Here's how the part is built. I have some questions about the finished solid (model axes, mm). A direction names the side the tool comes from. Round coordinates to 2 decimals unless told otherwise and drop trailing zeros. Write each loop counter-clockwise with the first axis right and the second up, starting at its lowest first coordinate (ties: lowest second). Pieces come first, ordered by that corner, then holes. Notation, with made-up numbers: (18, 79.25) -> (51, 79.25) arc R24 cw to (51, 115.25) -> close; hole circle Ø3 at (25.5, 65.5). An arc over 180 degrees is marked (long way). Answer in a Markdown table with one row per item.
from build123d import *

# Parameters (mm, degrees)
BOSS_EXTRUDE1_DEPTH = 7
FILLET1_R           = 2
SKETCH2_R           = 1.5
SKETCH2_R_2         = 1.1
BOSS_EXTRUDE2_DEPTH = 4
SKETCH3_R           = 1.5
SKETCH3_R_2         = 1.1
SKETCH3_W           = 4.5
SKETCH3_H           = 1.5
BOSS_EXTRUDE3_DEPTH = 4


with BuildPart() as part:
    # Sketch1 → Boss-Extrude1 (new body)
    with BuildSketch(Plane(origin=(0, 0, 0), x_dir=(1, 0, 0), z_dir=(0, 1, 0))):
        with BuildLine():
            Line((10, 9), (-10, 9))
            ThreePointArc((-10, 9), (-11.414213562, 8.414213562), (-12, 7))
            Line((-12, 7), (-12, -7))
            ThreePointArc((-12, -7), (-11.414213562, -8.414213562), (-10, -9))
            Line((-10, -9), (10, -9))
            ThreePointArc((10, -9), (11.414213562, -8.414213562), (12, -7))
            Line((12, -7), (12, 7))
            ThreePointArc((12, 7), (11.414213562, 8.414213562), (10, 9))
        make_face()
    extrude(amount=BOSS_EXTRUDE1_DEPTH)

    # Fillet1
    fillet1_edges = [part.edges().sort_by_distance(p)[0] for p in [
        (12, 0, 0),
        (11.414213562, 0, 8.414213562),
        (0, 0, 9),
        (-11.414213562, 0, 8.414213562),
        (11.414213562, 7, 8.414213562),
        (12, 7, 0),
        (11.414213562, 7, -8.414213562),
        (0, 7, -9),
        (-11.414213562, 7, -8.414213562),
        (-12, 7, 0),
        (-11.414213562, 7, 8.414213562),
        (-12, 0, 0),
        (0, 7, 9),
        (-11.414213562, 0, -8.414213562),
        (0, 0, -9),
        (11.414213562, 0, -8.414213562),
    ]]
    fillet(fillet1_edges, radius=FILLET1_R)

    # Sketch2 → Boss-Extrude2 (add)
    # profile 1 of 3: a face of its own
    with BuildSketch(Plane.ZY.offset(12)):
        with Locations(Location((0, 3.5, 0), (0, 0, 270))):
            Circle(SKETCH2_R)
        with Locations((0, 3.5)):
            Circle(SKETCH2_R_2, mode=Mode.SUBTRACT)
    # profile 2 of 3: a face of its own
    with BuildSketch(Plane.ZY.offset(12)):
        with Locations(Location((7, 3.5, 0), (0, 0, 270))):
            Circle(SKETCH2_R)
        with Locations(Location((7, 3.5, 0), (0, 0, 90))):
            Circle(SKETCH2_R_2, mode=Mode.SUBTRACT)
    # profile 3 of 3: a face of its own
    with BuildSketch(Plane.ZY.offset(12)):
        with Locations(Location((-7, 3.5, 0), (0, 0, 270))):
            Circle(SKETCH2_R)
        with Locations(Location((-7, 3.5, 0), (0, 0, 90))):
            Circle(SKETCH2_R_2, mode=Mode.SUBTRACT)
    extrude(amount=BOSS_EXTRUDE2_DEPTH)

    # Sketch3 → Boss-Extrude3 (add)
    # profile 1 of 3: a face of its own
    with BuildSketch(Plane(origin=(12, 0, 0), x_dir=(0, 0, -1), z_dir=(1, 0, 0))):
        with Locations(Location((-5.233431742, 3.5, 0), (0, 0, 270))):
            Circle(SKETCH3_R)
        with Locations((-5.233431742, 3.5)):
            Circle(SKETCH3_R_2, mode=Mode.SUBTRACT)
    # profile 2 of 3: a face of its own
    with BuildSketch(Plane(origin=(12, 0, 0), x_dir=(0, 0, -1), z_dir=(1, 0, 0))):
        with Locations(Location((-0.833431742, 3.5, 0), (0, 0, 270))):
            Circle(SKETCH3_R)
        with Locations((-0.833431742, 3.5)):
            Circle(SKETCH3_R_2, mode=Mode.SUBTRACT)
    # profile 3 of 3: a face of its own
    with BuildSketch(Plane(origin=(12, 0, 0), x_dir=(0, 0, -1), z_dir=(1, 0, 0))):
        with Locations((5.52417795, 3.5)):
            Rectangle(SKETCH3_W, SKETCH3_H)
    extrude(amount=BOSS_EXTRUDE3_DEPTH)


solid = part.part
1) I want a section at B-B, the plane z = 3.25. List the corners of the cut face in (x, y) for me, and give its area (3 significant figures).
Response:
| item | result |
|---|---|
| outline | (-12, 2) arc R2 ccw to (-10, 0) -> (10, 0) arc R2 ccw to (12, 2) -> (12, 5) arc R2 ccw to (10, 7) -> (-10, 7) arc R2 ccw to (-12, 5) -> close |
| area | 165 mm^2 |
2) I want a section at C-C, the plane x = 1.5. List the corners of the cut face in (y, z) for me.
Response:
| item | result |
|---|---|
| outline | (0, -7) arc R2 ccw to (2, -9) -> (5, -9) arc R2 ccw to (7, -7) -> (7, 7) arc R2 ccw to (5, 9) -> (2, 9) arc R2 ccw to (0, 7) -> close |
3) Which directions (+Z, -Z, +X, -X, +Y, -Y) give clear straight access to the entire face, cutting with the end or side of a thin tool? Please do faces 5 (the face through (14, 3, -7.774)), 6 (the face through (13.97, 4.59, 5.38)), 7 (the face through (-11.43, 0.6, 0.1)), 8 (the face through (0.14, 0.6, 8.43)), 9 (the face through (-12, 3.5, -6.6)).
Response:
| item | result |
|---|---|
| face 5 | -Z, +X, +Y, -Y |
| face 6 | +X |
| face 7 | +Z, -Z, -X, -Y |
| face 8 | +Z, +X, -X, -Y |
| face 9 | -X |
4) We'd pull the mould along Y, two halves only. Please class faces 1 (the face through (-11.43, 6.4, 0.1)), 2 (the face through (0, 3, -9)), 3 (the face through (13.97, 2.69, 3.97)), 4 (the face through (-13.97, 4.09, -7.93)): +Y half, -Y half, draft (parallel to the pull), parting line (faces both ways), or undercut.
Response:
| item | result |
|---|---|
| face 1 | +Y half |
| face 2 | draft |
| face 3 | parting line |
| face 4 | undercut |
5) I want a section at D-D, the plane y = 3.5. Count the separate pieces of the cut face and the enclosed holes in it, and give its area (3 significant figures).
Response:
| item | result |
|---|---|
| separate pieces | 3 |
| enclosed holes | 0 |
| area | 463 mm^2 |
6) I want a section at A-A, the plane x = 13. List the corners of the cut face in (y, z) for me.
Response:
| item | result |
|---|---|
| outline | circle Ø3 at (3.5, 0.83); circle Ø3 at (3.5, 5.23); (2.75, -7.77) -> (4.25, -7.77) -> (4.25, -3.27) -> (2.75, -3.27) -> close; hole circle Ø2.2 at (3.5, 0.83); hole circle Ø2.2 at (3.5, 5.23) |
7) For pin 1 (1.5 mm diameter, centred on y = 3, z = -2, fed in from +X); pin 2 (1.5 mm diameter, centred on y = 4, z = 2.5, fed in from -X); pin 3 (0.8 mm diameter, centred on x = 14, y = 3.5, fed in from -Z), each with a flat end and sliding along its axis, tell me the tip position at first contact or that it passes through.
Response:
| item | result |
|---|---|
| pin 1 | stops at x = 12 |
| pin 2 | stops at x = -12 |
| pin 3 | stops at z = -7.77 |
8) I need wall thicknesses on line 1 (X direction, y = 2.5, z = -6.25); line 2 (X direction, y = 4.25, z = 8); line 3 (X direction, y = 2.25, z = -1.25). Which ranges of each line are inside material? Lowest first, please. Write a range as [from, to].
Response:
| item | result |
|---|---|
| line 1 | x = [-16, 12] |
| line 2 | x = [-16, -12], [-11.73, 11.73] |
| line 3 | x = [-12, 12] |
